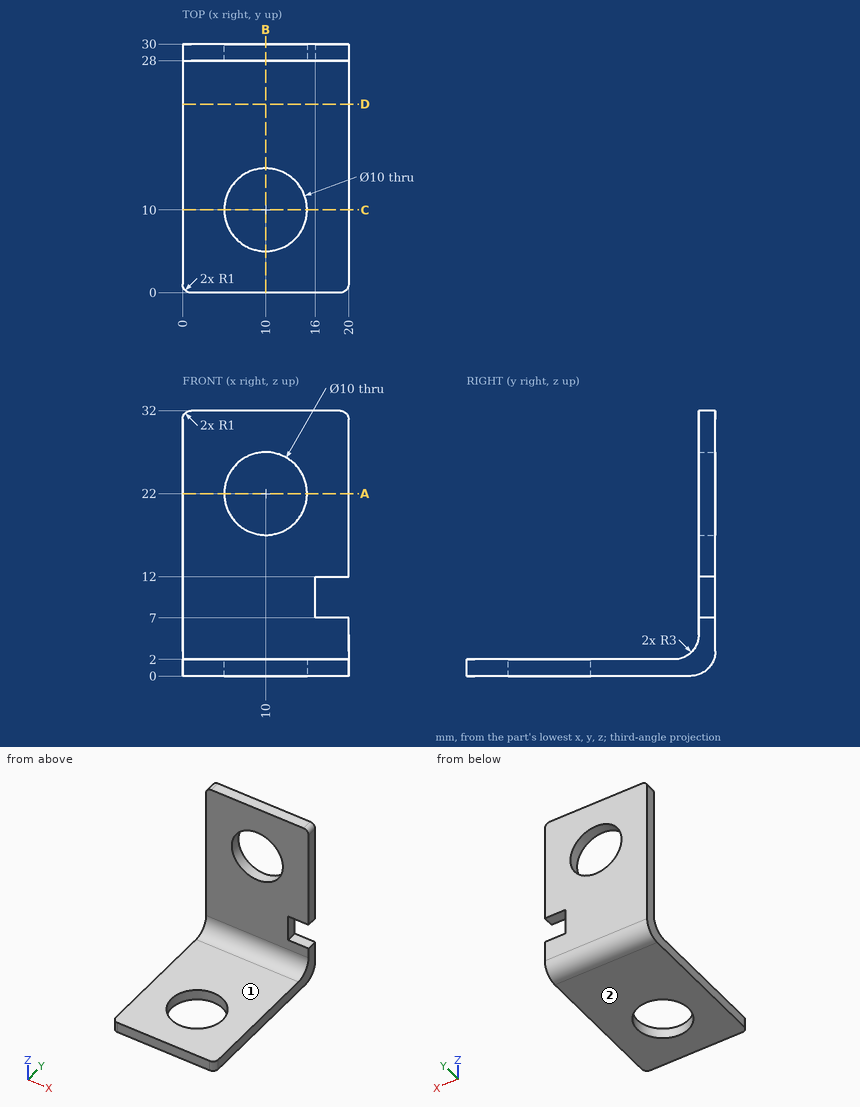
Print and shaded views of the part. All mm, measured from the part's lowest x, y and z. A direction names the side the tool comes from. Give positions to 0.01 mm unless a question says otherwise; leave off trailing zeros. Write each loop counter-clockwise with the first axis right and the second up, starting at its lowest first coordinate (ties: lowest second). Pieces come first, ordered by that corner, then holes. Notation, with made-up numbers: (1.25, -19) - (50.25, -19) arc R27 ccw to (50.25, 17) - close; hole circle Ø7 at (23, 6.5). An arc over 180 degrees is marked (long way). Put each result on its own line as item: value.
(1) Saw through at A-A (z = 22). List the corners of the cut face in (x, y).
Working result:
outline: (0, 28) - (5, 28) - (5, 30) - (0, 30) - close; (15, 28) - (20, 28) - (20, 30) - (15, 30) - close
(2) Tool access for the marked faces 1 and 2: list every direction of +Z, -Z, +X, -X, +Y, -Y with a clear straight run to the whole face (end or side of a thin tool).
Working result:
face 1: +Z, +X, -X, -Y
face 2: -Z, +X, -X, +Y, -Y
(3) Saw through at D-D (y = 22.75). List the corners of the cut face in (x, z), then the cut area to 3 significant figures.
Working result:
outline: (0, 0) - (20, 0) - (20, 2) - (0, 2) - close
area: 40.0 mm^2
(4) Drop flat-ended pins along their axis: pin 1 Ø10 at (y, z) = (23.5, 23) entering from -X; pin 2 Ø11.5 at (x, y) = (10, 10) entering from +Z; pin 3 Ø1 at (y, z) = (29.5, 9) entering from +X; pin 4 Ø1 at (x, y) = (17.5, 29.5) entering from -Z. Give the stop position or say it passes through.
Working result:
pin 1: x = 0
pin 2: z = 2
pin 3: x = 16
pin 4: z = 0.76
(5) Saw through at B-B (x = 10). List the corners of the cut face in (y, z).
Working result:
outline: (0, 0) - (5, 0) - (5, 2) - (0, 2) - close; (15, 0) - (27, 0) arc R3 ccw to (30, 3) - (30, 17) - (28, 17) - (28, 5) arc R3 cw to (25, 2) - (15, 2) - close; (28, 27) - (30, 27) - (30, 32) - (28, 32) - close
(6) Wall check: L1, parallel to Y at x = 8.5, z = 17; L2, parallel to Z at x = 10.25, y = 17.25; L3, parallel to Y at x = 10, z = 0.4. Give the ranges that are in metal, low to high.
Working result:
L1: 28 to 30
L2: 0 to 2
L3: 0 to 5, 15 to 28.5
(7) Saw through at C-C (y = 10). List the corners of the cut face in (x, z).
Working result:
outline: (0, 0) - (5, 0) - (5, 2) - (0, 2) - close; (15, 0) - (20, 0) - (20, 2) - (15, 2) - close
